from build123d import *

# Parameters (mm, degrees)
SKETCH1_R           = 2
BOSS_EXTRUDE2_DEPTH = 24
BOSS_EXTRUDE3_START = -14
BOSS_EXTRUDE3_DEPTH = 14


with BuildPart() as part:
    # Sketch1 → Boss-Extrude2 (new body)
    with BuildSketch(Plane.XY):
        Circle(SKETCH1_R)
    extrude(amount=BOSS_EXTRUDE2_DEPTH)

    # Sketch1<4> → Boss-Extrude3 (add)
    with BuildSketch(Plane.XY.offset(BOSS_EXTRUDE3_START)):
        with BuildLine():
            Line((1.322875656, 1.5), (-1.322875656, 1.5))
            ThreePointArc((-1.322875656, 1.5), (-0.822875656, -1.822875656), (2, 0))
            ThreePointArc((2, 0), (1.822875656, 0.822875656), (1.322875656, 1.5))
        make_face()
    extrude(amount=BOSS_EXTRUDE3_DEPTH)


solid = part.part
Build history of the part. All positions in model axes, mm. A direction names the side the tool comes from. Coordinates: 2 decimals unless noted, no trailing zeros. Order: outer loops, then holes, each group sorted by start corner. A loop starts at its lowest first (then second) coordinate and runs counter-clockwise, first axis right, second up. Notation, with made-up numbers: (-37, -29.75) - (-6, -29.75) arc R27 ccw to (-6, -5.75) - close; hole circle Ø6 at (62.5, -21.5). An arc over 180 degrees is marked (long way). Write each question's results on one line, items separated by ' | '. Start each with the question number.
Item 1: Tool access for faces 1 (the face through (0, 0, -14)), 2 (the face through (0, 1.5, -7)): list every direction of +Z, -Z, +X, -X, +Y, -Y with a clear straight run to the whole face (end or side of a thin tool).
Item 2: Flat gauge pins, fed straight in: pin 1 (2 mm diameter, centred on y = 0.5, z = 16.5, fed in from -X); pin 2 (2 mm diameter, centred on x = 0.5, z = -9, fed in from +Y). Where does each tip first touch, or does it go through?
Item 3: Band-saw the part on B-B on z = -5. Write the cut outline in (x, y).
Item 4: Band-saw the part on C-C on z = 1.5. Write the cut outline in (x, y), and give its area (3 significant figures).
Item 5: Wall check: probe 1 along X at (y, z) = (-0.15, 19.5); probe 2 along Y at (x, z) = (1.5, 14); probe 3 along Y at (x, z) = (-0.25, -9). Give the ranges that are in metal, low to high. Write a range as [from, to].
Item 6: Band-saw the part on A-A on x = 0. Write the cut outline in (y, z), and give its area (3 significant figures).
Numbers:
1) face 1: -Z, +X, -X, +Y, -Y | face 2: -Z, +X, -X, +Y
2) pin 1: x = -2 | pin 2: y = 1.5
3) outline: (-1.32, 1.5) arc R2 ccw (long way) to (1.32, 1.5) - close
4) outline: circle Ø4 at (0, 0) | area: 12.6 mm^2
5) probe 1: [-1.99, 1.99] | probe 2: [-1.32, 1.32] | probe 3: [-1.98, 1.5]
6) outline: (-2, -14) - (1.5, -14) - (1.5, 0) - (2, 0) - (2, 24) - (-2, 24) - close | area: 145 mm^2
